Autodesk Inventor part; units mm, degrees
ref_plane "YZ Plane" through (0, 0, 0) normal (1, 0, 0) x (0, 1, 0)
ref_plane "XZ Plane" through (0, 0, 0) normal (0, 1, 0) x (-1, 0, 0)
ref_plane "XY Plane" through (0, 0, 0) normal (0, 0, 1) x (1, 0, 0)
sketch "Sketch1" plane through (0, 0, 0) normal (0, 0, 1) x (1, 0, 0)
  line L0 (0, 0) -> (-25.4, 0)
  line L1 (-25.4, 0) -> (-25.4, 25.4)
  line L2 (0, 3.175) -> (-22.225, 3.175)
  line L3 (-22.225, 3.175) -> (-22.225, 25.4)
  line L4 (-22.225, 25.4) -> (-25.4, 25.4)
  line L5 (0, 3.175) -> (0, 0)
  dimension "d0" = 25.4
  dimension "d1" = 25.4
  dimension "d2" = 3.175
extrude "Extrusion1" add sketch "Sketch1" along normal mid plane 819.15
properties part number "32.25 Top L w holes"
Check sheet for the modelled part. Datum: model origin and axes. Units: mm. A direction names the side the tool comes from. Coordinates: 2 decimals unless noted, no trailing zeros. Write each loop counter-clockwise with the first axis right and the second up, starting at its lowest first coordinate (ties: lowest second). Pieces come first, ordered by that corner, then holes. Notation, with made-up numbers: M 18,88.25 L 75,88.25 A25 cw 75,106.25 Z; hole C 25.5,86.25 d7. An arc over 180 degrees is marked long. Write item = value, one per line. Start each with the question number.
1. Go/stop test with flat-tipped pins: pin 1 (6.5 mm diameter, centred on x = -10, z = 147, fed in from +Y) (3 decimals); pin 2 (12 mm diameter, centred on y = 7, z = -13.5, fed in from +X). Record where each tip stops, or that it passes through.
2. Sectioned sample at A-A (z = 175). Record the cut outline in (x, y) (3 decimals).
3. Sectioned sample at C-C (y = 16). Record the cut outline in (x, z) (3 decimals).
4. Thickness scan on probe 1 along X at (y, z) = (13, -361.5) (3 decimals); probe 2 along Y at (x, z) = (-12, -99) (3 decimals). Record the ranges inside material, lowest first.
5. Tool access check on faces 1 (the flat face through (-22.225, 14, -6)), 2 (the flat face through (-18, 2, 409.575)). Record the directions out of +Z, -Z, +X, -X, +Y, -Y that give a thin tool (end or side, any length) a straight path to the whole face; none if there is none.
6. Sectioned sample at B-B (x = -7.75). Record the cut outline in (y, z) (3 decimals), then the cut area to 3 significant figures.
The answers:
q1.pin_1 = 3.175
q1.pin_2 = 0
q2.outline = M -25.4,0 L 0,0 L 0,3.175 L -22.225,3.175 L -22.225,25.4 L -25.4,25.4 Z
q3.outline = M -25.4,-409.575 L -22.225,-409.575 L -22.225,409.575 L -25.4,409.575 Z
q4.probe_1 = -25.4 to -22.225
q4.probe_2 = 0 to 3.175
q5.face_1 = +Z, -Z, +X, +Y
q5.face_2 = +Z, +X, -X, +Y, -Y
q6.outline = M 0,-409.575 L 3.175,-409.575 L 3.175,409.575 L 0,409.575 Z
q6.area = 2,600 mm²
